Source: CAD feature listing. Evaluate the final solid. Frame: model axes, mm. Give positions to 0.01 mm unless a question says otherwise; leave off trailing zeros. Loops run counter-clockwise (first coordinate to the right, second up) from the corner with the lowest first, then second, coordinate; pieces in that order, holes last. Notation, with made-up numbers: M 12.25,17.5 L 61.25,17.5 A37 ccw 61.25,56.5 Z; hole C 73.25,-7 d9. An arc over 180 degrees is marked long. Write item = value, one per line.
from build123d import *

# Parameters (mm, degrees)
FILLET2_R       = 0.2
SKETCH2_W       = 8.5
SKETCH2_H       = 1.2
SLOT_DEPTH      = 1.3
THDSCHPAT_COUNT = 19
THDSCHPAT_PITCH = 0.8


with BuildPart() as part:
    # BodySke → Base-Revolve (revolve)
    with BuildSketch(Plane.XY):
        Polygon((3.3, 2.5), (3.3, 4.25), (0, 3.96128741), (0, 0), (19.3, 0), (19.3, 2.5), align=None)
    revolve(axis=Axis((-25.4, 0, 0), (1, 0, 0)))

    # Fillet2
    fillet2_edges = [part.edges().sort_by_distance(p)[0] for p in [
        (0, -3.96128741, 0),
    ]]
    fillet(fillet2_edges, radius=FILLET2_R)

    # Sketch2 → Slot (cut)
    with BuildSketch(Plane(origin=(0, 0, 0), x_dir=(0, 0, -1), z_dir=(1, 0, 0))):
        Rectangle(SKETCH2_W, SKETCH2_H)
    extrude(amount=SLOT_DEPTH, mode=Mode.SUBTRACT)

    # ThdSchSke → ThreadSchematic (revolve, cut)
    with BuildSketch(Plane.XY):
        Polygon((4.9, -2.055), (4.588407645, -2.5), (4.588407645, -3.125), (5.211592355, -3.125), (5.211592355, -2.5), align=None)
    threadschematic = revolve(axis=Axis((-3.175, 0, 0), (1, 0, 0)), mode=Mode.SUBTRACT)

    # ThdSchPat: ThreadSchematic ×19
    with Locations(*[(i * THDSCHPAT_PITCH, 0, 0) for i in range(1, THDSCHPAT_COUNT)]):
        add(threadschematic, mode=Mode.SUBTRACT)


solid = part.part
1. Material intervals for probe 1 along X at (y, z) = (-0.25, 1.5); probe 2 along X at (y, z) = (-1.75, -3); probe 3 along Y at (x, z) = (1.25, 1), sorted ascending. Write a range as from..to.
Derived:
probe_1 = 1.3..19.3
probe_2 = 0..3.3
probe_3 = -3.95..-0.6, 0.6..3.95
2. First-contact query: pin 1 Ø4 at (x, y) = (11.5, 0.5) entering from -Z; pin 2 Ø0.6 at (y, z) = (0, 0) entering from -X; pin 3 Ø1 at (x, z) = (0.5, 0) entering from +Y. Flat tips, straight axial feed; report the tip coordinate or a pass-through.
Derived:
pin_1 = -2.5
pin_2 = 1.3
pin_3 = 4.05
3. Cut plane A-A, the plane x = 2. Return the cut outline in (y, z).
Derived:
outline = C 0,0 d8.27
4. Pull-direction query (X, two-part tool) for faces 1 (the flat face through (0, -2, 0)), 2 (the flat face through (19.3, 0, 0)), 3 (the cylindrical face through (3.94, -0.54, -2.44)); classes: +X half, -X half, draft (parallel to the pull), parting line (faces both ways), or undercut.
Derived:
face_1 = -X half
face_2 = +X half
face_3 = draft
